Build history of the part. All positions in model axes, mm. A direction names the side the tool comes from. Coordinates: 2 decimals unless noted, no trailing zeros. Order: outer loops, then holes, each group sorted by start corner. A loop starts at its lowest first (then second) coordinate and runs counter-clockwise, first axis right, second up. Notation, with made-up numbers: (24.5, 55) - (64.5, 55) arc R21 ccw to (64.5, 88) - close; hole circle Ø2 at (14.25, -34.5). An arc over 180 degrees is marked (long way). Answer as CSV lines item,"result". Start each with the question number.
from build123d import *

# Parameters (mm, degrees)
BOSS_EXTRUDE1_DEPTH     = 279.4
CONVERT_SOLID1_START    = -279.4
CONVERT_SOLID1_DEPTH    = 558.8
CONVERT_SOLID1_2_DEPTH  = 558.8
CUT_EXTRUDE1_DEPTH      = 586.091506768
EDGE_FLANGE1_DEPTH      = 412.817360463
EDGE_FLANGE1_BEND_DEPTH = 412.817360463
CUT_EXTRUDE2_DEPTH      = 588.256983898
CUT_EXTRUDE2_DEPTH_BACK = 588.256983898
SKETCH12_R              = 7.9375


# Read off the part's stored shape, not the designer's step: Convert-Solid1
# Sheet-metal steps are written as plain solids
with BuildPart() as part:
    # Sketch3 → Boss-Extrude1 (new, symmetric)
    with BuildSketch(Plane(origin=(0, 0, 0), x_dir=(0, 0, -1), z_dir=(1, 0, 0))):
        Polygon((-477.990419123, 101.6), (-503.390419123, 101.6), (-503.390419123, 104.14), (-477.723454365, 104.14), (-118.969509086, 27.884494906), (-119.497604781, 25.4), align=None)
    extrude(amount=BOSS_EXTRUDE1_DEPTH, both=True)

    # Convert-Solid1 outline → Convert-Solid1 (cut)
    with BuildSketch(Plane.YZ.offset(CONVERT_SOLID1_START)):
        with BuildLine():
            Line((104.14, 477.723454365), (104.14, 478.257383881))
            ThreePointArc((104.14, 478.257383881), (104.112171228, 477.726379287), (104.028989812, 477.201192491))
            Line((104.028989812, 477.201192491), (104.14, 477.723454365))
        make_face()
    extrude(amount=CONVERT_SOLID1_DEPTH, mode=Mode.SUBTRACT)

    # Convert-Solid1 2 outline → Convert-Solid1 2 (add)
    with BuildSketch(Plane.YZ.offset(CONVERT_SOLID1_START)):
        with BuildLine():
            Line((101.6, 477.990419123), (101.6, 478.257383881))
            ThreePointArc((101.6, 478.257383881), (101.586085614, 477.991881584), (101.544494906, 477.729288186))
            Line((101.544494906, 477.729288186), (101.6, 477.990419123))
        make_face()
    extrude(amount=CONVERT_SOLID1_2_DEPTH)

    # Sketch8 → Cut-Extrude1 (cut, through all)
    with BuildSketch(Plane(origin=(0, 2.484494906, -0.528095695), x_dir=(1, 0, 0), z_dir=(0, 0.9781476007338071, -0.2079116908177526))):
        Polygon((279.4, -488.402044668), (88.9, -122.167252357), (279.4, -122.167252357), align=None)
        Polygon((-88.9, -122.167252357), (-279.4, -488.402044668), (-279.4, -122.167252357), align=None)
    extrude(amount=-CUT_EXTRUDE1_DEPTH, mode=Mode.SUBTRACT)

    # Edge-Flange1 section (across the edge) → Edge-Flange1 (add)
    with BuildSketch(Plane(origin=(91.153384818, 25.156303297, 118.351101933), x_dir=(-0.8871593769725213, 0.09594358400127492, 0.4513790741037053), z_dir=(0.4614631511288068, 0.18445080609118078, 0.8677728160541709))):
        with BuildLine():
            Line((-2.54, 2.54), (-2.54, 22.86))
            Line((-2.54, 22.86), (0, 22.86))
            Line((0, 22.86), (0, 2.54))
            ThreePointArc((0, 2.54), (0.743948776, 0.743948776), (2.54, 0))
            Line((2.54, 0), (2.54, -2.54))
            ThreePointArc((2.54, -2.54), (-1.052102448, -1.052102448), (-2.54, 2.54))
        make_face()
    extrude(amount=EDGE_FLANGE1_DEPTH)

    # Edge-Flange1 section 2 (across the edge) → Edge-Flange1 bend (add)
    with BuildSketch(Plane(origin=(-281.653384818, 101.300798203, 476.582785338), x_dir=(0.8871593769725281, 0.09594358400127215, 0.45137907410369243), z_dir=(0.4614631511287936, -0.18445080609118217, -0.8677728160541774))):
        with BuildLine():
            Line((-2.54, 2.54), (-2.54, 22.86))
            Line((-2.54, 22.86), (0, 22.86))
            Line((0, 22.86), (0, 2.54))
            ThreePointArc((0, 2.54), (0.743948776, 0.743948776), (2.54, 0))
            Line((2.54, 0), (2.54, -2.54))
            ThreePointArc((2.54, -2.54), (-1.052102448, -1.052102448), (-2.54, 2.54))
        make_face()
    extrude(amount=EDGE_FLANGE1_BEND_DEPTH)

    # Sketch12 → Cut-Extrude2 (cut, two sides: drawn at the far end of the back side and taken through both)
    with BuildSketch(Plane(origin=(0, 2.484494906, -0.528095695), x_dir=(1, 0, 0), z_dir=(0, 0.9781476007338071, -0.2079116908177526)).offset(-CUT_EXTRUDE2_DEPTH_BACK)):
        with Locations((-20.371926238, 129.188925745)):
            Circle(SKETCH12_R)
        with Locations((120.282042226, -141.217252357)):
            Circle(SKETCH12_R)
    cut_extrude2 = extrude(amount=CUT_EXTRUDE2_DEPTH + CUT_EXTRUDE2_DEPTH_BACK, mode=Mode.SUBTRACT)

    # Mirror8: Cut-Extrude2 across plane
    add(cut_extrude2.mirror(Plane(origin=(0, 0, 0), x_dir=(0, 0, 1), z_dir=(1, 0, 0))), mode=Mode.SUBTRACT)


solid = part.part
(1) Probe L1, parallel to Y at x = 194.5, z = 465; L2, parallel to X at y = 51.5, z = 333; L3, parallel to X at y = 21, z = 160. List the from-to ranges inside material, lowest first. Write a range as [from, to].
(2) Pull direction X, two halves, no side cores. Call faces 1 (the flat face through (4, 101.6, 491)), 2 (the flat face through (-189.99, 51.23, 301.44)), 3 (the cylindrical face through (184.43, 62.02, 295.45)): +X half, -X half, draft (parallel to the pull), parting line (faces both ways), or undercut.
(3) Band-saw the part on B-B on y = 14.5. List the corners of the cut face in (x, z), plus the area to 3 significant figures.
(4) Drop flat-ended pins along their axis: pin 1 Ø8 at (y, z) = (43, 274.5) entering from +X; pin 2 Ø20 at (x, z) = (-113, 486) entering from -Y; pin 3 Ø4 at (x, y) = (67.5, 22.5) entering from +Z; pin 4 Ø2 at (y, z) = (103, 489.5) entering from -X. Give the stop position or say it passes through.
(5) Which spindle directions (+Z, -Z, +X, -X, +Y, -Y) get a long thin tool onto all of the face, cutting with end or side? Do faces 4 (the flat face through (3.91, 71.4, 335.91)), 5 (the flat face through (187.32, 50.17, 296.42)), 6 (the flat face through (185.07, 50.13, 297.63)). Say none if no direction does.
(6) Band-saw the part on A-A on x = -70. List the corners of the cut face in (y, z), plus the area to 3 significant figures.
Filled in:
1,L1,"y = [98.84, 101.44]"
1,L2,"x = [-206.08, -203.21], [203.21, 206.08]"
1,L3,"x = [-114.76, -111.89], [111.89, 114.76]"
2,face 1,"draft"
2,face 2,"-X half"
2,face 3,"undercut"
3,outline,"(-123.3, 178.17) - (-93.41, 119.42) - (-91.15, 120.62) - (-120.44, 178.17) - close; (91.15, 120.62) - (93.41, 119.42) - (123.3, 178.17) - (120.44, 178.17) - close"
3,area,"333 mm^2"
4,pin 1,"stops at x = 177.47"
4,pin 2,"stops at y = 101.18"
4,pin 3,"passes through"
4,pin 4,"stops at x = -279.4"
5,face 4,"+Z, -Y"
5,face 5,"-Z, +X, -Y"
5,face 6,"+Z"
6,outline,"(25.4, 119.5) - (27.88, 118.97) - (104.03, 477.2) arc R5.08 ccw to (104.14, 478.26) - (104.14, 503.39) - (101.6, 503.39) - (101.6, 478.26) arc R2.54 cw to (101.54, 477.73) - close"
6,area,"996 mm^2"
